```python
from build123d import *

# Parameters (mm, degrees)
F0_W     = 50.8
F0_H     = 63.5
F1_DEPTH = 31.75
F3_DEPTH = 31.751
F5_DEPTH = 19.05
F6_R     = 3.175
F7_DEPTH = 25.4
F8_R     = 6.35
F9_DEPTH = 31.751


with BuildPart() as f1:
    # F0 (on Front) → F1 (new body)
    with BuildSketch(Plane.XZ):
        with Locations((-43.838402, 38.215244)):
            Rectangle(F0_W, F0_H)
    extrude(amount=F1_DEPTH)

    # F2 (on face) → F3 (cut, through all)
    with BuildSketch(Plane(origin=(0, 0, 0), x_dir=(-1, 0, 0), z_dir=(0, 1, 0))):
        with BuildLine():
            Line((18.438402, 69.965244), (18.438402, 12.815244))
            ThreePointArc((18.438402, 12.815244), (27.418658, 16.534988), (31.138402, 25.515244))
            Line((31.138402, 25.515244), (31.138402, 57.265244))
            ThreePointArc((31.138402, 57.265244), (34.858146, 66.2455), (43.838402, 69.965244))
            Line((43.838402, 69.965244), (18.438402, 69.965244))
        make_face()
        with BuildLine():
            ThreePointArc((56.538402, 25.515244), (60.258146, 16.534988), (69.238402, 12.815244))
            Line((69.238402, 12.815244), (69.238402, 69.965244))
            Line((69.238402, 69.965244), (43.838402, 69.965244))
            ThreePointArc((43.838402, 69.965244), (52.818658, 66.2455), (56.538402, 57.265244))
            Line((56.538402, 57.265244), (56.538402, 25.515244))
        make_face()
    extrude(amount=-F3_DEPTH, mode=Mode.SUBTRACT)

    # F4 (on face) → F5 (cut)
    with BuildSketch(Plane.XZ.offset(31.75)):
        with BuildLine():
            ThreePointArc((-56.538402, 25.515244), (-60.258146, 16.534988), (-69.238402, 12.815244))
            Line((-69.238402, 12.815244), (-18.438402, 12.815244))
            ThreePointArc((-18.438402, 12.815244), (-27.418658, 16.534988), (-31.138402, 25.515244))
            Line((-31.138402, 25.515244), (-31.138402, 57.265244))
            ThreePointArc((-31.138402, 57.265244), (-43.838402, 44.565244), (-56.538402, 57.265244))
            Line((-56.538402, 57.265244), (-56.538402, 25.515244))
        make_face()
    extrude(amount=-F5_DEPTH, mode=Mode.SUBTRACT)

    # F6 (on face) → F7 (cut)
    with BuildSketch(Plane.XY.offset(12.815244)):
        with Locations((-27.963402, -22.225)):
            Circle(F6_R)
        with Locations((-59.713402, -22.225)):
            Circle(F6_R)
        with BuildLine():
            Line((-69.238402, -31.75), (-59.713402, -31.75))
            ThreePointArc((-59.713402, -31.75), (-66.448594, -28.960192), (-69.238402, -22.225))
            Line((-69.238402, -22.225), (-69.238402, -31.75))
        make_face()
        with BuildLine():
            ThreePointArc((-18.438402, -22.225), (-21.22821, -28.960192), (-27.963402, -31.75))
            Line((-27.963402, -31.75), (-18.438402, -31.75))
            Line((-18.438402, -31.75), (-18.438402, -22.225))
        make_face()
    extrude(amount=-F7_DEPTH, mode=Mode.SUBTRACT)

    # F8 (on face) → F9 (cut, through all)
    with BuildSketch(Plane.XZ.offset(31.75)):
        with Locations((-43.83729, 57.265244)):
            Circle(F8_R)
    extrude(amount=-F9_DEPTH, mode=Mode.SUBTRACT)


solid = f1.part
```
Verification items for the finished model (mm, model axes). A direction names the side the tool comes from. Coordinates: 2 decimals unless noted, no trailing zeros. Loops run counter-clockwise (first coordinate to the right, second up) from the corner with the lowest first, then second, coordinate; pieces in that order, holes last. Notation, with made-up numbers: (-24, 29.5) - (25, 29.5) arc R7 ccw to (25, 42.5) - close; hole circle Ø3 at (27.25, 44). An arc over 180 degrees is marked (long way). Answer as a JSON object with one key per item and string values.
(1) Cross-section at A-A, the plane y = -17.5. Record the boundary of the cut face in (x, z), then the cut area to 3 significant figures.
Response:
{"outline": "(-69.24, 6.47) - (-18.44, 6.47) - (-18.44, 12.82) - (-69.24, 12.82) - close; circle Ø25.4 at (-43.84, 57.27); hole circle Ø12.7 at (-43.84, 57.27)", "area": "703 mm²"}
(2) Scan lines: line 1 along Y through (x, z) = (-36, 24); line 2 along Z through (x, y) = (-47.5, -18.5); line 3 along Z through (x, y) = (-63, -25). Record each from-to range of solid material in increasing order.
Response:
{"line 1": "y = -12.7 to 0", "line 2": "z = 6.47 to 12.82, 45.1 to 52.08, 62.45 to 69.43", "line 3": "z = 6.47 to 12.82"}
(3) Mould release check, pull along Z, two halves, no side actions. Record for faces 4 (the flat face through (-44, 0, 32)), 5 (the flat face through (-44, -16, 6.465)), 6 (the flat face through (-44, -22, 12.815)): pulls with the +Z half, pulls with the -Z half, needs draft (parallel to the pull), parting line crosses it, or undercut.
Response:
{"face 4": "needs draft", "face 5": "pulls with the -Z half", "face 6": "undercut"}
(4) Go/stop test with flat-tipped pins: pin 1 Ø14 at (y, z) = (-7.5, 41) entering from -X; pin 2 Ø10 at (x, z) = (-46, 23) entering from -Y; pin 3 Ø4 at (y, z) = (-5.5, 39) entering from +X. Record where each tip stops, or that it passes through.
Response:
{"pin 1": "stops at x = -56.54", "pin 2": "stops at y = -12.7", "pin 3": "stops at x = -31.14"}
(5) Access from +Z, -Z, +X, -X, +Y, -Y to the whole of each face (thin tool, end or side, straight path). Record for faces 1 (the flat face through (-31.138, -6, 41)), 2 (the cylindrical face through (-44.66, -16.1, 63.56)), 3 (the flat face through (-56.538, -6, 42)).
Response:
{"face 1": "+Z, +X, +Y, -Y", "face 2": "+Y, -Y", "face 3": "+Z, -X, +Y, -Y"}
(6) Cross-section at D-D, the plane z = 54.5. Record the boundary of the cut face in (x, y).
Response:
{"outline": "(-56.54, -12.7) - (-56.23, -12.7) - (-56.23, -31.75) - (-49.55, -31.75) - (-49.55, 0) - (-56.54, 0) - close; (-38.12, -31.75) - (-31.44, -31.75) - (-31.44, -12.7) - (-31.14, -12.7) - (-31.14, 0) - (-38.12, 0) - close"}
(7) Cross-section at B-B, the plane x = -47.5. Record the boundary of the cut face in (y, z), then the cut area to 3 significant figures.
Response:
{"outline": "(-31.75, 6.47) - (0, 6.47) - (0, 52.08) - (-31.75, 52.08) - (-31.75, 45.1) - (-12.7, 45.1) - (-12.7, 12.82) - (-31.75, 12.82) - close; (-31.75, 62.45) - (0, 62.45) - (0, 69.43) - (-31.75, 69.43) - close", "area": "1,050 mm²"}
(8) Cross-section at C-C, the plane y = -21. Record the boundary of the cut face in (x, z), then the cut area to 3 significant figures.
Response:
{"outline": "(-69.24, 6.47) - (-62.64, 6.47) - (-62.64, 12.82) - (-69.24, 12.82) - close; (-56.78, 6.47) - (-30.89, 6.47) - (-30.89, 12.82) - (-56.78, 12.82) - close; circle Ø25.4 at (-43.84, 57.27); (-25.03, 6.47) - (-18.44, 6.47) - (-18.44, 12.82) - (-25.03, 12.82) - close; hole circle Ø12.7 at (-43.84, 57.27)", "area": "628 mm²"}
